Work out the finished part from the listing and answer in its coordinate system (mm). Face numbers are marked on the shaded views. A direction names the side the tool comes from. Give positions to 0.01 mm unless a question says otherwise; leave off trailing zeros. Loops run counter-clockwise (first coordinate to the right, second up) from the corner with the lowest first, then second, coordinate; pieces in that order, holes last. Notation, with made-up numbers: (-34.75, -29.5) - (-12.75, -29.5) arc R20 ccw to (-12.75, -21.5) - close; hole circle Ø3 at (80.25, 43). An arc over 180 degrees is marked (long way). One line per question, with ' | ' between items.
from build123d import *

# Parameters (mm, degrees)
F0_W     = 2.38125
F0_H     = 12.7
F1_DEPTH = 9.525
F3_D     = 3.2004
F5_D     = 5.1054
F5_DEPTH = 9.271
F5_TIP   = 1.5338169022


with BuildPart() as f1:
    # F0 (on Front) → F1 (new body)
    with BuildSketch(Plane.XZ):
        Polygon((0, -9.525), (0, 0), (-2.38125, 0), (-4.7625, 0), (-4.7625, -9.525), align=None)
        Polygon((2.38125, 0), (0, 0), (0, -9.525), (4.7625, -9.525), (4.7625, 0), align=None)
        with Locations((1.190625, 6.35)):
            Rectangle(F0_W, F0_H)
        with Locations((-1.190625, 6.35)):
            Rectangle(F0_W, F0_H)
    extrude(amount=F1_DEPTH)

    # F3 (through all)
    with Locations(Plane.YZ.offset(2.38125)):
        with Locations((-4.7625, 7.9375)):
            Hole(F3_D / 2)

    # F5
    with Locations(Plane(origin=(0, 0, -9.525), x_dir=(1, 0, 0), z_dir=(0, 0, -1))):
        with Locations((0, 4.7625)):
            Hole(F5_D / 2, depth=F5_DEPTH)
            with Locations((0, 0, -(F5_DEPTH + F5_TIP / 2))):  # 118° drill point
                Cone(0, F5_D / 2, F5_TIP, mode=Mode.SUBTRACT)


solid = f1.part
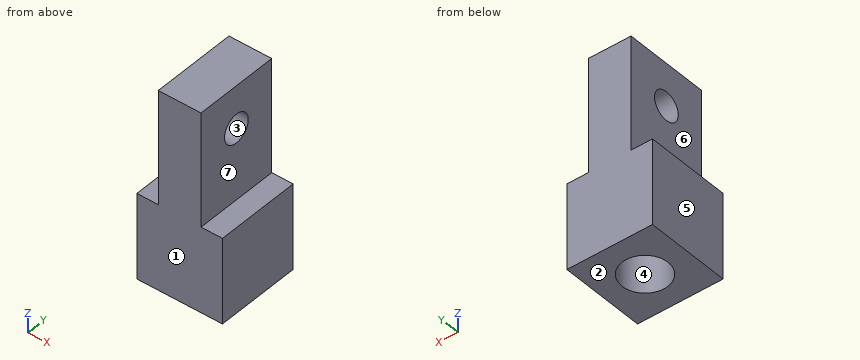
1. Find section B-B on y = -8. Write down the section's boundary in (x, z) (1 decimal), then the cut area to 3 significant figures.
Evaluation:
outline: (-4.8, -9.5) - (4.8, -9.5) - (4.8, 0) - (2.4, 0) - (2.4, 12.7) - (-2.4, 12.7) - (-2.4, 0) - (-4.8, 0) - close | area: 151 mm2
2. Find section A-A on z = -5. Write down the section's boundary in (x, y) (1 decimal), then the cut area to 3 significant figures.
Evaluation:
outline: (-4.8, -9.5) - (4.8, -9.5) - (4.8, 0) - (-4.8, 0) - close; hole circle Ø5.1 at (0, -4.8) | area: 70.3 mm2
3. Which of the six approach directions +Z, -Z, +X, -X, +Y, -Y give full straight-line access (tool end or side, diameter ignored) to the marked faces 5, 6 and 7?
Evaluation:
face 5: +Z, -Z, -X, +Y, -Y | face 6: +Z, -X, +Y, -Y | face 7: +Z, +X, +Y, -Y
4. Consider L1, parallel to X at y = -3.75, z = 10; L2, parallel to Y at x = 0, z = -5.5 (3 decimals); L3, parallel to Z at x = -2.5, y = -8.75 (3 decimals). Determine where each line is inside the solid, lowest interval first.
Evaluation:
L1: -2.38 to 2.38 | L2: -9.525 to -7.315, -2.21 to 0 | L3: -9.525 to 0
5. Find section C-C on z = 2.5. Write down the section's boundary in (x, y) (3 decimals).
Evaluation:
outline: (-2.381, -9.525) - (2.381, -9.525) - (2.381, 0) - (-2.381, 0) - close
6. Determine the mould class of the marked faces 1, 2, 3 and 4 for opening direction Y: +Y half, -Y half, draft (parallel to the pull), parting line (faces both ways), or undercut.
Evaluation:
face 1: -Y half | face 2: draft | face 3: undercut | face 4: undercut
7. Flat-ended cylindrical pins translate along their axes: pin 1 (5 mm diameter, centred on y = -4, z = 6.5, fed in from +X); pin 2 (1.2 mm diameter, centred on x = 3.5, y = -5, fed in from +Z). Find the tip coordinate at first contact, or state that the pin passes through.
Evaluation:
pin 1: x = 2.38 | pin 2: z = 0
